Design review of the part built by this model. Coordinates are the model's own, in mm. A direction names the side the tool comes from. Give positions to 0.01 mm unless a question says otherwise; leave off trailing zeros. Write each loop counter-clockwise with the first axis right and the second up, starting at its lowest first coordinate (ties: lowest second). Pieces come first, ordered by that corner, then holes.
Autodesk Inventor part; units mm, degrees
ref_plane "rod_cp_XY" through (0, 0, 0) normal (1, 0, 0) x (0, 0, -1)
ref_plane "rod_cp_YZ" through (0, 0, 0) normal (0, 0, -1) x (0, 1, 0)
ref_plane "rod_cp_ZX" through (0, 0, 0) normal (0, 1, 0) x (1, 0, 0)
sketch "Sketch_1" plane through (0, 0, 0) normal (0, 0, 1) x (1, 0, 0)
  line L0 (163.5252, 0) -> (0, 0)
  line L1 (0, 0) -> (0, 3.175)
  line L2 (0, 3.175) -> (142.0876, 3.175)
  line L3 (142.0876, 3.175) -> (142.0876, 9.6203)
  line L4 (142.0876, 9.6203) -> (163.5252, 9.6203)
  line L5 (163.5252, 9.6203) -> (163.5252, 0)
  line L6 (163.5252, 0) -> (0, 0)
revolve "Revolution1" add sketch "Sketch_1" angle 360 about axis through (163.5252, 0, 0) along (1, 0, 0)
sketch "Sketch_3" plane through (0, 0, 0) normal (0, 0, 1) x (1, 0, 0)
  line L0 (0, 0) -> (-12.7, 0)
  line L1 (-12.7, 0) -> (-12.7, 2.634)
  line L2 (-12.7, 2.634) -> (-12.159, 3.175)
  line L3 (-12.159, 3.175) -> (0, 3.175)
  line L4 (0, 3.175) -> (0, 0)
  line L5 (0, 0) -> (-12.7, 0)
revolve "Revolution2" add sketch "Sketch_3" angle 360 about axis through (0, 0, 0) along (1, 0, 0)
thread "Thread1"
sketch "Sketch_30" plane through (0, 0, 0) normal (0, 0, 1) x (1, 0, 0)
  line L0 (0, 0) -> (-0.254, 0)
  line L1 (-0.254, 3.429) -> (-0.254, 2.921)
  line L2 (-0.254, 2.921) -> (0, 2.921)
  line L3 (0, 2.921) -> (0, 3.429)
  line L4 (0, 3.429) -> (-0.254, 3.429)
revolve "Revolution3" cut sketch "Sketch_30" angle 360 about axis through (0, 0, 0) along (1, 0, 0)
ref_plane "rod_cp_XY" through (0, 0, 0) normal (1, 0, 0) x (0, 0, -1)
ref_plane "rod_cp_YZ" through (0, 0, 0) normal (0, 0, -1) x (0, 1, 0)
ref_plane "rod_cp_ZX" through (0, 0, 0) normal (0, 1, 0) x (1, 0, 0)
ref_plane "to_rod_clevis_XY" through (-12.7, 0, 0) normal (1, 0, 0) x (0, 0, -1)
ref_plane "to_rod_clevis_YZ" through (-12.7, 0, 0) normal (0, 0, -1) x (0, 1, 0)
ref_plane "to_rod_clevis_ZX" through (-12.7, 0, 0) normal (0, 1, 0) x (1, 0, 0)
ref_plane "rl2_XY" through (0, 0, 0) normal (1, 0, 0) x (0, 0, -1)
ref_plane "rl2_YZ" through (0, 0, 0) normal (0, 0, -1) x (0, 1, 0)
ref_plane "rl2_ZX" through (0, 0, 0) normal (0, 1, 0) x (1, 0, 0)
ref_plane "rl1_XY" through (-12.7, 0, 0) normal (1, 0, 0) x (0, 0, -1)
ref_plane "rl1_YZ" through (-12.7, 0, 0) normal (0, 0, -1) x (0, 1, 0)
ref_plane "rl1_ZX" through (-12.7, 0, 0) normal (0, 1, 0) x (1, 0, 0)
ref_plane "thd1_XY" through (-12.7, 3.175, 0) normal (1, 0, 0) x (0, 0, -1)
ref_plane "thd1_YZ" through (-12.7, 3.175, 0) normal (0, 0, -1) x (0, 1, 0)
ref_plane "thd1_ZX" through (-12.7, 3.175, 0) normal (0, 1, 0) x (1, 0, 0)
ref_plane "thd2_XY" through (-12.7, -3.175, 0) normal (1, 0, 0) x (0, 0, -1)
ref_plane "thd2_YZ" through (-12.7, -3.175, 0) normal (0, 0, -1) x (0, 1, 0)
ref_plane "thd2_ZX" through (-12.7, -3.175, 0) normal (0, 1, 0) x (1, 0, 0)
ref_plane "dia1_XY" through (0, 3.175, 0) normal (1, 0, 0) x (0, 0, -1)
ref_plane "dia1_YZ" through (0, 3.175, 0) normal (0, 0, -1) x (0, 1, 0)
ref_plane "dia1_ZX" through (0, 3.175, 0) normal (0, 1, 0) x (1, 0, 0)
ref_plane "dia2_XY" through (0, -3.175, 0) normal (1, 0, 0) x (0, 0, -1)
ref_plane "dia2_YZ" through (0, -3.175, 0) normal (0, 0, -1) x (0, 1, 0)
ref_plane "dia2_ZX" through (0, -3.175, 0) normal (0, 1, 0) x (1, 0, 0)
ref_plane "hh1_XY" through (193.6496, 0, 0) normal (0, 0, 1) x (1, 0, 0)
ref_plane "hh1_YZ" through (193.6496, 0, 0) normal (1, 0, 0) x (0, 1, 0)
ref_plane "hh1_ZX" through (193.6496, 0, 0) normal (0, 1, 0) x (0, 0, 1)
ref_plane "hh2_XY" through (200.0504, 0, 0) normal (0, 0, 1) x (1, 0, 0)
ref_plane "hh2_YZ" through (200.0504, 0, 0) normal (1, 0, 0) x (0, 1, 0)
ref_plane "hh2_ZX" through (200.0504, 0, 0) normal (0, 1, 0) x (0, 0, 1)
ref_plane "dia12_XY" through (0, 0, 10.9537) normal (1, 0, 0) x (0, 0, -1)
ref_plane "dia12_YZ" through (0, 0, 10.9537) normal (0, 0, -1) x (0, 1, 0)
ref_plane "dia12_ZX" through (0, 0, 10.9537) normal (0, 1, 0) x (1, 0, 0)
ref_plane "dia22_XY" through (0, 0, -10.9537) normal (1, 0, 0) x (0, 0, -1)
ref_plane "dia22_YZ" through (0, 0, -10.9537) normal (0, 0, -1) x (0, 1, 0)
ref_plane "dia22_ZX" through (0, 0, -10.9537) normal (0, 1, 0) x (1, 0, 0)
properties part number "044-DXP0_rod"
(1) To check wall thickness, follow L1, parallel to Z at x = 103.5, y = 0 (3 decimals); L2, parallel to X at y = 0.5, z = -7; L3, parallel to Z at x = 101.5, y = 1.5. State the ranges of each line that lie inside material, in increasing order.
Resolved:
L1: z = -3.175 to 3.175
L2: x = 142.09 to 163.53
L3: z = -2.8 to 2.8
(2) Consider section D-D, the plane y = 7.5. Give the boundary of the cut face in (x, z).
Resolved:
outline: (142.09, -6.02) - (163.53, -6.02) - (163.53, 6.02) - (142.09, 6.02) - close
(3) Consider section A-A, the plane z = 0. Give the boundary of the cut face in (x, y) (3 decimals).
Resolved:
outline: (-12.7, -2.634) - (-12.159, -3.175) - (-0.254, -3.175) - (-0.254, -2.921) - (0, -2.921) - (0, -3.175) - (142.088, -3.175) - (142.088, -9.62) - (163.525, -9.62) - (163.525, 9.62) - (142.088, 9.62) - (142.088, 3.175) - (0, 3.175) - (0, 2.921) - (-0.254, 2.921) - (-0.254, 3.175) - (-12.159, 3.175) - (-12.7, 2.634) - close
(4) Clearance check with flat-ended pins moving along their axes: P1, Ø1.5, axis at y = 2, z = -6, coming from the -X side; P2, Ø10, axis at x = 37.5, z = -6, coming from the -Y side; P3, Ø2, axis at x = 58, z = 3, coming from the +Y side. State where each tip first meets the part, or that it passes through.
Resolved:
P1: stops at x = 142.09
P2: stops at y = -3.01
P3: stops at y = 2.47
(5) Tool access review of faces 1 (the face through (72.04, -0.69, -3.1)), 2 (the face through (152.96, -2.09, -9.39)): name each direction out of +Z, -Z, +X, -X, +Y, -Y from which nothing blocks a thin tool from reaching the whole face with its end or side.
Resolved:
face 1: -X
face 2: +X, -X
(6) Consider section C-C, the plane x = 56. Give the boundary of the cut face in (y, z) (3 decimals), then the cut area to 3 significant figures.
Resolved:
outline: circle Ø6.35 at (0, 0)
area: 31.7 mm2
